```python
from build123d import *

# Parameters (mm, degrees)
SKETCH1_R           = 25
SKETCH1_R_2         = 12.5
SKETCH1_R_3         = 28
SKETCH1_R_4         = 16
BOSS_EXTRUDE1_DEPTH = 35


with BuildPart() as part:
    # Sketch1 → Boss-Extrude1 (new, symmetric)
    # profile 1 of 3: a face of its own
    with BuildSketch(Plane.XY):
        with BuildLine():
            ThreePointArc((-25, 12.609520213), (0, 28), (25, 12.609520213))
            Line((25, 12.609520213), (25, 110))
            ThreePointArc((25, 110), (0, 85), (-25, 110))
            Line((-25, 110), (-25, 92))
            Line((-25, 92), (-25, 12.609520213))
        make_face()
    # profile 2 of 3: a face of its own
    with BuildSketch(Plane.XY):
        with Locations((0, 110)):
            Circle(SKETCH1_R)
        with Locations((0, 110)):
            Circle(SKETCH1_R_2, mode=Mode.SUBTRACT)
    # profile 3 of 3: a face of its own
    with BuildSketch(Plane.XY):
        Circle(SKETCH1_R_3)
        Circle(SKETCH1_R_4, mode=Mode.SUBTRACT)
    extrude(amount=BOSS_EXTRUDE1_DEPTH, both=True)


solid = part.part
```
Design review of the part built by this model. Coordinates are the model's own, in mm. A direction names the side the tool comes from. Coordinates: 2 decimals unless noted, no trailing zeros. Write each loop counter-clockwise with the first axis right and the second up, starting at its lowest first coordinate (ties: lowest second). Pieces come first, ordered by that corner, then holes.
1) Machinability: for faces 1 (the flat face through (0, 55, -35)), 2 (the flat face through (25, 61, 0)), which of the approach directions +Z, -Z, +X, -X, +Y, -Y give a long, thin tool a straight path to every point of the face, cutting with its end or side? Answer none if there is none.
2) Insertion check: pin 1 (6 mm diameter, centred on x = -11.5, z = 4, fed in from -Y); pin 2 (4 mm diameter, centred on x = 3.5, z = -26.5, fed in from +Y); pin 3 (1.5 mm diameter, centred on x = 20, z = 21.5, fed in from +Y). Each pin has a flat end and moves straight along its axis. Give the tip position at first contact, or say it passes through.
3) Add section B-B (y = 0). Write out the cut boundary in (x, z), plus the area to 3 significant figures.
4) Add section D-D (y = 58). Write out the cut boundary in (x, z).
5) Add section C-C (z = 24). Write out the cut boundary in (x, y), plus the area to 3 significant figures.
6) To check wall thickness, follow L1, parallel to Y at x = 0, z = 27; L2, parallel to Y at x = 10, z = -18; L3, parallel to X at y = 68.5, z = -23.5. State the ranges of each line that lie inside material, in increasing order.
7) Add section A-A (x = 0). Write out the cut boundary in (y, z), plus the area to 3 significant figures.
Check result:
1. face 1: -Z, +X, -X, +Y, -Y
1. face 2: +Z, -Z, +X, +Y
2. pin 1: stops at y = -26.68
2. pin 2: stops at y = 134.95
2. pin 3: stops at y = 125.95
3. outline: (-28, -35) - (-16, -35) - (-16, 35) - (-28, 35) - close; (16, -35) - (28, -35) - (28, 35) - (16, 35) - close
3. area: 1,680 mm2
4. outline: (-25, -35) - (25, -35) - (25, 35) - (-25, 35) - close
5. outline: (-25, 12.61) arc R28 ccw (long way) to (25, 12.61) - (25, 110) arc R25 ccw to (-25, 110) - close; hole circle Ø32 at (0, 0); hole circle Ø25 at (0, 110)
5. area: 6,470 mm2
6. L1: y = -28 to -16, 16 to 97.5, 122.5 to 135
6. L2: y = -26.15 to -12.49, 12.49 to 102.5, 117.5 to 132.91
6. L3: x = -25 to 25
7. outline: (-28, -35) - (-16, -35) - (-16, 35) - (-28, 35) - close; (16, -35) - (97.5, -35) - (97.5, 35) - (16, 35) - close; (122.5, -35) - (135, -35) - (135, 35) - (122.5, 35) - close
7. area: 7,420 mm2
